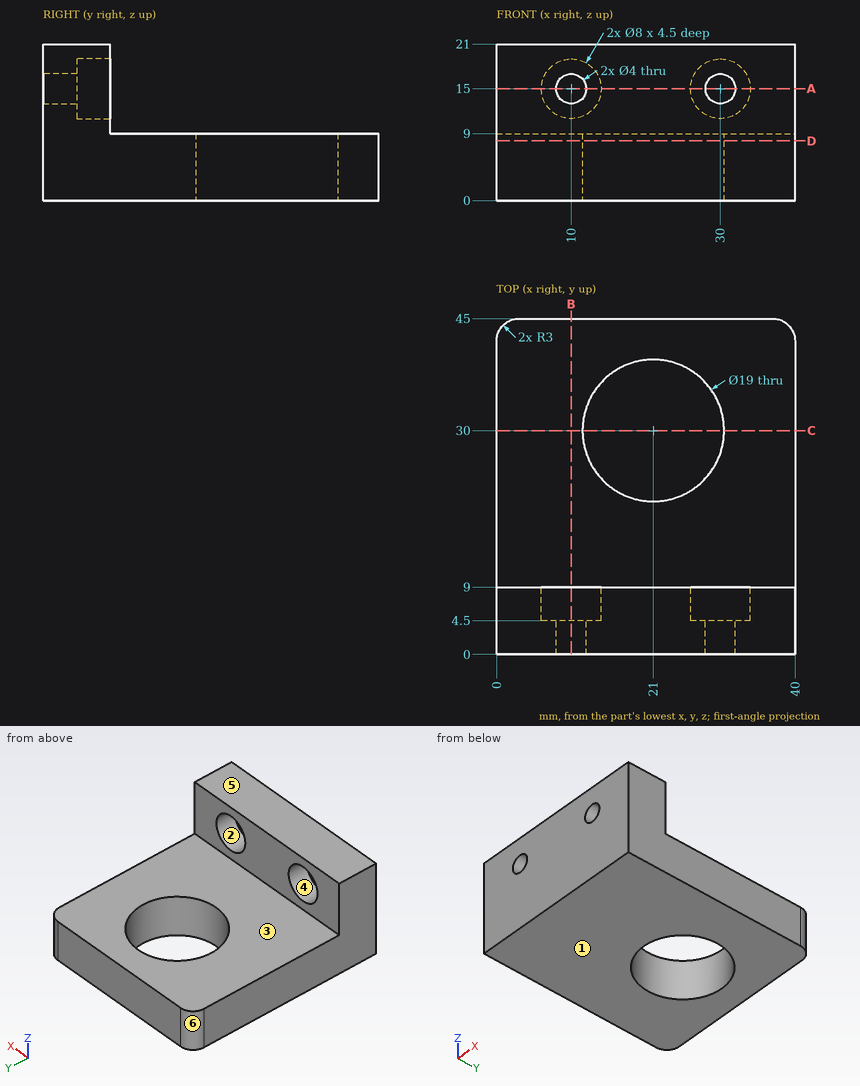
Print and shaded views of the part. All mm, measured from the part's lowest x, y and z. A direction names the side the tool comes from. Round coordinates to 2 decimals unless told otherwise and drop trailing zeros. Write each loop counter-clockwise with the first axis right and the second up, starting at its lowest first coordinate (ties: lowest second). Pieces come first, ordered by that corner, then holes.
Item 1: Which spindle directions (+Z, -Z, +X, -X, +Y, -Y) get a long thin tool onto all of the face, cutting with end or side? Do the marked faces 1, 2 and 3. Say none if no direction does.
Results:
face 1: -Z, +X, -X, +Y, -Y
face 2: +Y
face 3: +Z, +X, -X, +Y
Item 2: Two-plate mould, pull along X, no slides. Class the marked faces 4, 5 and 6: +X half, -X half, draft (parallel to the pull), parting line (faces both ways), or undercut.
Results:
face 4: undercut
face 5: draft
face 6: -X half
Item 3: Cut at D-D, the plane z = 8. Give the cut face in (x, y), plus the area to 3 significant figures.
Results:
outline: (0, 0) - (40, 0) - (40, 42) arc R3 ccw to (37, 45) - (3, 45) arc R3 ccw to (0, 42) - close; hole circle Ø19 at (21, 30)
area: 1,510 mm2
Item 4: Cut at C-C, the plane y = 30. Give the cut face in (x, z), plus the area to 3 significant figures.
Results:
outline: (0, 0) - (11.5, 0) - (11.5, 9) - (0, 9) - close; (30.5, 0) - (40, 0) - (40, 9) - (30.5, 9) - close
area: 189 mm2
Item 5: Cut at B-B, the plane x = 10. Give the cut face in (y, z).
Results:
outline: (0, 0) - (45, 0) - (45, 9) - (9, 9) - (9, 11) - (4.5, 11) - (4.5, 13) - (0, 13) - close; (0, 17) - (4.5, 17) - (4.5, 19) - (9, 19) - (9, 21) - (0, 21) - close
Item 6: Probe L1, parallel to X at y = 7.1, z = 15; L2, parallel to Z at x = 15.5, y = 43.5. List the from-to ranges inside material, lowest first.
Results:
L1: x = 0 to 6, 14 to 26, 34 to 40
L2: z = 0 to 9
Item 7: Cut at A-A, the plane z = 15. Give the cut face in (x, y), plus the area to 3 significant figures.
Results:
outline: (0, 0) - (8, 0) - (8, 4.5) - (6, 4.5) - (6, 9) - (0, 9) - close; (12, 0) - (28, 0) - (28, 4.5) - (26, 4.5) - (26, 9) - (14, 9) - (14, 4.5) - (12, 4.5) - close; (32, 0) - (40, 0) - (40, 9) - (34, 9) - (34, 4.5) - (32, 4.5) - close
area: 252 mm2
Item 8: Drop flat-ended pins along their axis: pin 1 Ø3.5 at (x, z) = (19, 13) entering from +Y; pin 2 Ø5 at (x, y) = (30, 10.5) entering from -Z; pin 3 Ø2.5 at (x, z) = (8.5, 13) entering from +Y; pin 4 Ø8 at (x, y) = (34, 34) entering from +Z. Give the stop position or say it passes through.
Results:
pin 1: stops at y = 9
pin 2: stops at z = 0
pin 3: stops at y = 4.5
pin 4: stops at z = 9
